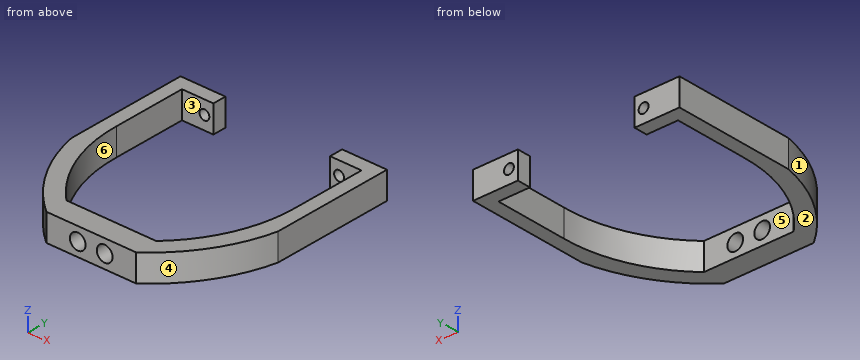
from build123d import *

# Parameters (mm, degrees)
CYLINDER001_R     = 1.75
CYLINDER001_DEPTH = 10
CYLINDER002_R     = 1.1
CYLINDER002_DEPTH = 10
CYLINDER003_R     = 1.1
CYLINDER003_DEPTH = 10
CYLINDER_R        = 1.75
CYLINDER_DEPTH    = 10
EXTRUDE_DEPTH     = 6


with BuildPart() as cylinder001:
    # Cylinder001 → Cylinder001 (new body)
    with BuildSketch(Plane(origin=(-3, -7, 3), x_dir=(1, 0, 0), z_dir=(0, 1, 0))):
        Circle(CYLINDER001_R)
    extrude(amount=CYLINDER001_DEPTH)


with BuildPart() as cylinder002:
    # Cylinder002 → Cylinder002 (new body)
    with BuildSketch(Plane(origin=(15, 43, 3), x_dir=(1, 0, 0), z_dir=(0, -1, 0))):
        Circle(CYLINDER002_R)
    extrude(amount=CYLINDER002_DEPTH)


with BuildPart() as cylinder003:
    # Cylinder003 → Cylinder003 (new body)
    with BuildSketch(Plane(origin=(-15, 43, 3), x_dir=(1, 0, 0), z_dir=(0, -1, 0))):
        Circle(CYLINDER003_R)
    extrude(amount=CYLINDER003_DEPTH)


with BuildPart() as fusion:
    # Cylinder → Cylinder (new body)
    with BuildSketch(Plane(origin=(3, -7, 3), x_dir=(1, 0, 0), z_dir=(0, 1, 0))):
        Circle(CYLINDER_R)
    extrude(amount=CYLINDER_DEPTH)

    # Fusion: union Cylinder001, Cylinder002, Cylinder003
    add(cylinder001.part)
    add(cylinder002.part)
    add(cylinder003.part)


with BuildPart() as cut:
    # Sketch → Extrude (new body)
    with BuildSketch(Plane.XY):
        with BuildLine():
            Line((-13, 40), (-13, 43))
            Line((-13, 43), (-23, 43))
            Line((-23, 43), (-23, 15.823169))
            ThreePointArc((-23, 15.823169), (-18.331197, 4.268359), (-10, -5))
            Line((-10, -5), (10, -5))
            ThreePointArc((10, -5), (18.331197, 4.268359), (23, 15.823169))
            Line((23, 43), (23, 15.823169))
            Line((13, 43), (23, 43))
            Line((13, 40), (13, 43))
            Line((13, 40), (20, 40))
            Line((20, 40), (20, 23.620741))
            ThreePointArc((10, 0), (17.454834, 10.7711), (20, 23.620741))
            Line((-10, 0), (10, 0))
            ThreePointArc((-20, 23.620741), (-17.454834, 10.7711), (-10, 0))
            Line((-20, 40), (-20, 23.620741))
            Line((-13, 40), (-20, 40))
        make_face()
    extrude(amount=EXTRUDE_DEPTH)

    # Cut: cut Fusion
    add(fusion.part, mode=Mode.SUBTRACT)


solid = cut.part
The listing builds one solid part. Answer for the finished solid, in the listing's coordinates (mm). Face numbers are marked on the shaded views. A direction names the side the tool comes from. Give positions to 0.01 mm unless a question says otherwise; leave off trailing zeros. Write each loop counter-clockwise with the first axis right and the second up, starting at its lowest first coordinate (ties: lowest second). Pieces come first, ordered by that corner, then holes. Notation, with made-up numbers: (71.5, -38) -> (122.5, -38) arc R20 cw to (122.5, -11) -> close; hole circle Ø4 at (10.5, 79). An arc over 180 degrees is marked (long way). One line per question, with ' | ' between items. Start each with the question number.
1. Section B-B (x = -3) is taken. Determine the outline of the cut face in (y, z), plus the area to 3 significant figures.
2. For a pull along Y with two mould halves and no side action, classify the marked faces 1, 2 and 3 as pulls with the +Y half, pulls with the -Y half, needs draft (parallel to the pull), parting line crosses it, or undercut.
3. Section C-C (z = 3) is taken. State how many separate pieces and enclosed holes the cut face has, plus the area to 3 significant figures.
4. Section D-D (z = 5.4) is taken. Determine the outline of the cut face in (x, y), plus the area to 3 significant figures.
5. Find the intervals of material crossed by probe 1 along X at (y, z) = (32.5, 1.45); probe 2 along Z at (x, y) = (-3, -3); probe 3 along X at (y, z) = (41.8, 3), in increasing order.
6. Section A-A (y = 28.5) is taken. Determine the outline of the cut face in (x, z).
7. Given pin 1 Ø1.8 at (x, z) = (15, 3) entering from +Y; pin 2 Ø3 at (x, z) = (2.5, 3.5) entering from +Y; pin 3 Ø3 at (y, z) = (12.5, 3) entering from -X, each flat-ended and moving along its own axis, determine where each tip first touches the part or whether it passes through.
8. For the marked faces 4, 5 and 6, determine the directions among +Z, -Z, +X, -X, +Y, -Y from which every point of the face is accessible in a straight line to the end or side of a thin tool.
Response values:
1) outline: (-5, 0) -> (0, 0) -> (0, 1.25) -> (-5, 1.25) -> close; (-5, 4.75) -> (0, 4.75) -> (0, 6) -> (-5, 6) -> close | area: 12.5 mm2
2) face 1: pulls with the -Y half | face 2: needs draft | face 3: undercut
3) separate pieces: 5 | enclosed holes: 0 | area: 426 mm2
4) outline: (-23, 15.82) arc R35.97 ccw to (-10, -5) -> (10, -5) arc R35.97 ccw to (23, 15.82) -> (23, 43) -> (13, 43) -> (13, 40) -> (20, 40) -> (20, 23.62) arc R32.18 cw to (10, 0) -> (-10, 0) arc R32.18 cw to (-20, 23.62) -> (-20, 40) -> (-13, 40) -> (-13, 43) -> (-23, 43) -> close | area: 475 mm2
5) probe 1: -23 to -20, 20 to 23 | probe 2: 0 to 1.25, 4.75 to 6 | probe 3: -23 to -16.1, -13.9 to -13, 13 to 13.9, 16.1 to 23
6) outline: (-23, 0) -> (-20, 0) -> (-20, 6) -> (-23, 6) -> close; (20, 0) -> (23, 0) -> (23, 6) -> (20, 6) -> close
7) pin 1: y = 7.6 | pin 2: y = 0 | pin 3: x = -22.56
8) face 4: +Z, -Z, +X, -Y | face 5: +Z, -Z, +Y | face 6: +Z, -Z
